Could you check a few things on this model? Use its own coordinates, in mm. Give positions to 0.01 mm unless a question says otherwise; leave off trailing zeros. Loops run counter-clockwise (first coordinate to the right, second up) from the corner with the lowest first, then second, coordinate; pieces in that order, holes last. Notation, with made-up numbers: (4.25, 21) - (17.25, 21) arc R19 ccw to (17.25, 41) - close; hole circle Ø1 at (-39, 35). An arc over 180 degrees is marked (long way). Use CSV: the item, a comma, the result in double quotes.
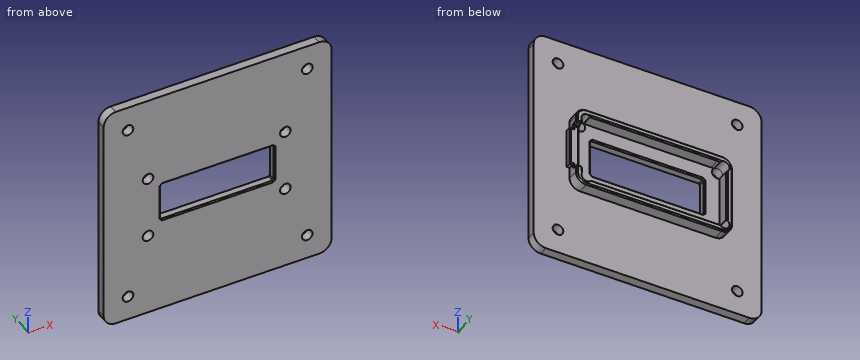
from build123d import *

# Parameters (mm, degrees)
SKETCH_1_W                      = 75
SKETCH_1_H                      = 75
SKETCH_1_R                      = 1.75
SKETCH_1_W_2                    = 37.4
SKETCH_1_H_2                    = 12.4
EXTRUDE_1_DEPTH                 = 3
SKETCH_2_W                      = 51.4
SKETCH_2_H                      = 26.4
SKETCH_2_W_2                    = 47.4
SKETCH_2_H_2                    = 22.4
EXTRUDE_2_DEPTH                 = 4
SKETCH_3_W                      = 2
SKETCH_3_H                      = 15.2
CUT_EXTRUDE_1_DEPTH             = 2
SKETCH_4_W                      = 1
SKETCH_4_H                      = 12.8
EXTRUDE_3_DEPTH                 = 2
FILLET_1_R                      = 2.8
FILLET_2_R                      = 3.4
CHAMFER_1_SIZE                  = 0.4
CUT_EXTRUDE_2_REACH             = 55.184
SKETCH_5_R                      = 1.75
CUT_EXTRUDE_2_DIRECTION_2_DEPTH = 54.183644102
FILLET_3_R                      = 4


with BuildPart() as part:
    # 草图1 → 凸台-拉伸1 (new body)
    with BuildSketch(Plane(origin=(0, 0, 0), x_dir=(1, 0, 0), z_dir=(0, 1, 0))):
        Rectangle(SKETCH_1_W, SKETCH_1_H)
        with Locations(Location((-29.5, 29.5, 0), (0, 0, 270))):
            Circle(SKETCH_1_R, mode=Mode.SUBTRACT)
        with Locations(Location((29.5, 29.5, 0), (0, 0, 270))):
            Circle(SKETCH_1_R, mode=Mode.SUBTRACT)
        with Locations(Location((29.5, -29.5, 0), (0, 0, 270))):
            Circle(SKETCH_1_R, mode=Mode.SUBTRACT)
        with Locations(Location((-29.5, -29.5, 0), (0, 0, 270))):
            Circle(SKETCH_1_R, mode=Mode.SUBTRACT)
        Rectangle(SKETCH_1_W_2, SKETCH_1_H_2, mode=Mode.SUBTRACT)
    extrude(amount=EXTRUDE_1_DEPTH)

    # 草图2 → 凸台-拉伸2 (add)
    with BuildSketch(Plane(origin=(0, 3, 0), x_dir=(1, 0, 0), z_dir=(0, 1, 0))):
        Rectangle(SKETCH_2_W, SKETCH_2_H)
        Rectangle(SKETCH_2_W_2, SKETCH_2_H_2, mode=Mode.SUBTRACT)
    extrude(amount=EXTRUDE_2_DEPTH)

    # 草图3 → 切除-拉伸1 (cut)
    with BuildSketch(Plane(origin=(0, 7, 0), x_dir=(1, 0, 0), z_dir=(0, 1, 0))):
        with Locations((24.7, -0.3)):
            Rectangle(SKETCH_3_W, SKETCH_3_H)
    extrude(amount=-CUT_EXTRUDE_1_DEPTH, mode=Mode.SUBTRACT)

    # 草图4 → 凸台-拉伸3 (add)
    with BuildSketch(Plane(origin=(0, 3, 0), x_dir=(1, 0, 0), z_dir=(0, 1, 0))):
        with Locations((26.2, -0.3)):
            Rectangle(SKETCH_4_W, SKETCH_4_H)
    extrude(amount=EXTRUDE_3_DEPTH)

    # 圆角1
    fillet_1_edges = [part.edges().sort_by_distance(p)[0] for p in [
        (23.7, 5, -11.2),
        (-23.7, 5, -11.2),
        (-23.7, 5, 11.2),
        (23.7, 5, 11.2),
    ]]
    fillet(fillet_1_edges, radius=FILLET_1_R)

    # 圆角2
    fillet_2_edges = [part.edges().sort_by_distance(p)[0] for p in [
        (25.7, 5, 13.2),
        (25.7, 5, -13.2),
        (-25.7, 5, -13.2),
        (-25.7, 5, 13.2),
    ]]
    fillet(fillet_2_edges, radius=FILLET_2_R)

    # 倒角1
    chamfer_1_edges = [part.edges().sort_by_distance(p)[0] for p in [
        (0, 7, 11.2),
        (23.7, 7, 8.15),
        (-23.7, 7, 0),
        (0, 7, -11.2),
        (22.879898987, 7, 10.379898987),
        (-22.879898987, 7, 10.379898987),
        (22.879898987, 7, -10.379898987),
        (-22.879898987, 7, -10.379898987),
        (0, 7, -13.2),
        (-25.7, 7, 0),
        (0, 7, 13.2),
        (25.7, 7, 8.85),
        (-24.704163056, 7, -12.204163056),
        (-24.704163056, 7, 12.204163056),
        (24.704163056, 7, 12.204163056),
        (24.704163056, 7, -12.204163056),
        (18.7, 0, 0),
        (18.7, 1.5, 6.2),
        (0, 0, -6.2),
        (18.7, 1.5, -6.2),
        (-18.7, 0, 0),
        (-18.7, 1.5, -6.2),
        (0, 0, 6.2),
        (-18.7, 1.5, 6.2),
        (18.7, 3, 0),
        (0, 3, -6.2),
        (-18.7, 3, 0),
        (0, 3, 6.2),
        (23.7, 7, -7.85),
        (25.7, 7, -8.55),
        (23.7, 5, 0.3),
        (23.7, 6, 7.9),
        (24.7, 5, -7.3),
        (23.7, 6, -7.3),
        (25.7, 5, 7.3),
        (25.7, 6, -7.3),
        (24.7, 5, 7.9),
        (25.7, 6, 7.9),
        (24.7, 7, 7.9),
        (24.7, 7, -7.3),
        (25.7, 5, -6.7),
        (26.2, 5, 6.7),
        (26.7, 5, 0.3),
        (26.2, 5, -6.1),
    ]]
    chamfer(chamfer_1_edges, length=CHAMFER_1_SIZE)

    # 草图5 → 切除-拉伸2 (cut, up to next)
    with BuildSketch(Plane(origin=(0, 3, 0), x_dir=(1, 0, 0), z_dir=(0, 1, 0)), mode=Mode.PRIVATE) as cut_extrude_2_sk1:
        with Locations(Location((-22.91, 10.4, 0), (0, 0, 40.156544446))):
            Circle(SKETCH_5_R)
    cut_extrude_2_tool1 = extrude(cut_extrude_2_sk1.sketch, amount=-CUT_EXTRUDE_2_REACH, mode=Mode.PRIVATE) & part.part
    # 草图5 → 切除-拉伸2 (cut, up to next)
    with BuildSketch(Plane(origin=(0, 3, 0), x_dir=(1, 0, 0), z_dir=(0, 1, 0)), mode=Mode.PRIVATE) as cut_extrude_2_sk2:
        with Locations(Location((22.3, 10.4, 0), (0, 0, 136.81614849))):
            Circle(SKETCH_5_R)
    cut_extrude_2_tool2 = extrude(cut_extrude_2_sk2.sketch, amount=-CUT_EXTRUDE_2_REACH, mode=Mode.PRIVATE) & part.part
    # 草图5 → 切除-拉伸2 (cut, up to next)
    with BuildSketch(Plane(origin=(0, 3, 0), x_dir=(1, 0, 0), z_dir=(0, 1, 0)), mode=Mode.PRIVATE) as cut_extrude_2_sk3:
        with Locations(Location((22.3, -9.8, 0), (0, 0, 37.891788933))):
            Circle(SKETCH_5_R)
    cut_extrude_2_tool3 = extrude(cut_extrude_2_sk3.sketch, amount=-CUT_EXTRUDE_2_REACH, mode=Mode.PRIVATE) & part.part
    # 草图5 → 切除-拉伸2 (cut, up to next)
    with BuildSketch(Plane(origin=(0, 3, 0), x_dir=(1, 0, 0), z_dir=(0, 1, 0)), mode=Mode.PRIVATE) as cut_extrude_2_sk4:
        with Locations(Location((-22.91, -9.8, 0), (0, 0, 116.835376612))):
            Circle(SKETCH_5_R)
    cut_extrude_2_tool4 = extrude(cut_extrude_2_sk4.sketch, amount=-CUT_EXTRUDE_2_REACH, mode=Mode.PRIVATE) & part.part
    add(cut_extrude_2_tool1.solids().sort_by_distance((-22.91, 3, -10.4))[0], mode=Mode.SUBTRACT)
    add(cut_extrude_2_tool2.solids().sort_by_distance((22.3, 3, -10.4))[0], mode=Mode.SUBTRACT)
    add(cut_extrude_2_tool3.solids().sort_by_distance((22.3, 3, 9.8))[0], mode=Mode.SUBTRACT)
    add(cut_extrude_2_tool4.solids().sort_by_distance((-22.91, 3, 9.8))[0], mode=Mode.SUBTRACT)

    # 草图5 → 切除-拉伸2 direction 2 (cut)
    with BuildSketch(Plane(origin=(0, 3, 0), x_dir=(1, 0, 0), z_dir=(0, 1, 0))):
        with Locations(Location((-22.91, 10.4, 0), (0, 0, 40.156544446))):
            Circle(SKETCH_5_R)
        with Locations(Location((22.3, 10.4, 0), (0, 0, 136.81614849))):
            Circle(SKETCH_5_R)
        with Locations(Location((22.3, -9.8, 0), (0, 0, 37.891788933))):
            Circle(SKETCH_5_R)
        with Locations(Location((-22.91, -9.8, 0), (0, 0, 116.835376612))):
            Circle(SKETCH_5_R)
    extrude(amount=CUT_EXTRUDE_2_DIRECTION_2_DEPTH, mode=Mode.SUBTRACT)

    # 圆角3
    fillet_3_edges = [part.edges().sort_by_distance(p)[0] for p in [
        (37.5, 1.5, 37.5),
        (-37.5, 1.5, 37.5),
        (-37.5, 1.5, -37.5),
        (37.5, 1.5, -37.5),
    ]]
    fillet(fillet_3_edges, radius=FILLET_3_R)


solid = part.part
1) Suppose I cut it at D-D (z = -29.5). Please give me the cut outline in (x, y).
Answer below:
outline,"(-37.5, 0) - (-31.25, 0) - (-31.25, 3) - (-37.5, 3) - close; (-27.75, 0) - (27.75, 0) - (27.75, 3) - (-27.75, 3) - close; (31.25, 0) - (37.5, 0) - (37.5, 3) - (31.25, 3) - close"
2) Suppose I cut it at C-C (x = 6.5). Please give me the cut outline in (y, z), plus the area to 3 significant figures.
Answer below:
outline,"(0, -37.5) - (3, -37.5) - (3, -13.2) - (6.6, -13.2) - (7, -12.8) - (7, -11.6) - (6.6, -11.2) - (3, -11.2) - (3, -6.6) - (2.6, -6.2) - (0.4, -6.2) - (0, -6.6) - close; (0, 6.6) - (0.4, 6.2) - (2.6, 6.2) - (3, 6.6) - (3, 11.2) - (6.6, 11.2) - (7, 11.6) - (7, 12.8) - (6.6, 13.2) - (3, 13.2) - (3, 37.5) - (0, 37.5) - close"
area,"203 mm2"
3) I need wall thicknesses on line 1 along Z through (x, y) = (22.3, 2.1); line 2 along X through (y, z) = (1.95, -10.4); line 3 along Z through (x, y) = (16, 0.75). Which ranges of each line are inside material? Lowest first, please.
Answer below:
line 1,"z = -37.5 to -12.15, -8.65 to 8.05, 11.55 to 37.5"
line 2,"x = -37.5 to -24.66, -21.16 to 20.55, 24.05 to 37.5"
line 3,"z = -37.5 to -6.2, 6.2 to 37.5"
4) Suppose I cut it at B-B (z = -4.5). Please give me the cut outline in (x, y), plus the area to 3 significant figures.
Answer below:
outline,"(-37.5, 0) - (-19.1, 0) - (-18.7, 0.4) - (-18.7, 2.6) - (-19.1, 3) - (-23.7, 3) - (-23.7, 6.6) - (-24.1, 7) - (-25.3, 7) - (-25.7, 6.6) - (-25.7, 3) - (-37.5, 3) - close; (18.7, 0.4) - (19.1, 0) - (37.5, 0) - (37.5, 3) - (26.7, 3) - (26.7, 4.6) - (26.3, 5) - (24.1, 5) - (23.7, 4.6) - (23.7, 3) - (19.1, 3) - (18.7, 2.6) - close"
area,"126 mm2"
5) Suppose I cut it at A-A (x = 29.5). Please give me the cut outline in (y, z).
Answer below:
outline,"(0, -37.5) - (3, -37.5) - (3, -31.25) - (0, -31.25) - close; (0, -27.75) - (3, -27.75) - (3, 27.75) - (0, 27.75) - close; (0, 31.25) - (3, 31.25) - (3, 37.5) - (0, 37.5) - close"
6) I'm going to push flat-ended pins straight in: P1, Ø0.8, axis at x = 26.5, y = 3.5, coming from the +Z side; P2, Ø1.8, axis at x = 2, y = 5, coming from the -Z side; P3, Ø0.8, axis at y = 4, z = 0, coming from the +X side. Where does each tip first touch, or does it pass through?
Answer below:
P1,"stops at z = 6.7"
P2,"stops at z = -13.2"
P3,"stops at x = 26.7"
